```python
from build123d import *

# Parameters (mm, degrees)
SKETCH1_R           = 2.125
BOSS_EXTRUDE1_DEPTH = 5.5
BOSS_EXTRUDE2_START = 7
SKETCH4_R           = 13.5
BOSS_EXTRUDE2_DEPTH = 7
SKETCH6_R           = 11
CUT_EXTRUDE4_DEPTH  = 4
SKETCH5_R           = 1
SKETCH5_R_2         = 1.75
CUT_EXTRUDE2_DEPTH  = 40.376388864
CHAMFER1_SIZE       = 2
SKETCH7_R           = 3
CUT_EXTRUDE5_DEPTH  = 3
FILLET1_R           = 1
SKETCH8_R           = 3
SKETCH8_R_2         = 2.125
BOSS_EXTRUDE3_DEPTH = 0.5
CUT_EXTRUDE6_DEPTH  = 3.25
FILLET2_R           = 0.5


with BuildPart() as part:
    # Sketch1 → Boss-Extrude1 (new body)
    with BuildSketch(Plane.XY):
        with BuildLine():
            Line((-13.071318793, 3.375), (-5.809475019, 31.5))
            ThreePointArc((-5.809475019, 31.5), (0, 36), (5.809475019, 31.5))
            Line((5.809475019, 31.5), (13.071318793, 3.375))
            ThreePointArc((13.071318793, 3.375), (0, -13.5), (-13.071318793, 3.375))
        make_face()
        with Locations((0, 30)):
            Circle(SKETCH1_R, mode=Mode.SUBTRACT)
    extrude(amount=BOSS_EXTRUDE1_DEPTH)

    # Sketch4 → Boss-Extrude2 (add)
    with BuildSketch(Plane(origin=(0, 0, 0), x_dir=(-1, 0, 0), z_dir=(0, 0, -1)).offset(BOSS_EXTRUDE2_START)):
        Circle(SKETCH4_R)
    extrude(amount=-BOSS_EXTRUDE2_DEPTH)

    # Sketch6 → Cut-Extrude4 (cut)
    with BuildSketch(Plane(origin=(0, 0, -7), x_dir=(-1, 0, 0), z_dir=(0, 0, -1))):
        Circle(SKETCH6_R)
    extrude(amount=-CUT_EXTRUDE4_DEPTH, mode=Mode.SUBTRACT)

    # Sketch5 → Cut-Extrude2 (cut, through all)
    with BuildSketch(Plane(origin=(0, 0, -3), x_dir=(-1, 0, 0), z_dir=(0, 0, -1))):
        with Locations((7.42, 0)):
            Circle(SKETCH5_R)
        with Locations((0, -7.42)):
            Circle(SKETCH5_R)
        with Locations((-7.42, 0)):
            Circle(SKETCH5_R)
        with Locations((0, 7.42)):
            Circle(SKETCH5_R)
        Circle(SKETCH5_R_2)
    extrude(amount=-CUT_EXTRUDE2_DEPTH, mode=Mode.SUBTRACT)

    # Chamfer1
    chamfer1_edges = [part.edges().sort_by_distance(p)[0] for p in [
        (9.440396906, 17.4375, 5.5),
        (0, 36, 5.5),
        (-9.440396906, 17.4375, 5.5),
        (0, -13.5, 5.5),
    ]]
    chamfer(chamfer1_edges, length=CHAMFER1_SIZE)

    # Sketch7 → Cut-Extrude5 (cut)
    with BuildSketch(Plane.XY.offset(5.5)):
        Circle(SKETCH7_R)
    extrude(amount=-CUT_EXTRUDE5_DEPTH, mode=Mode.SUBTRACT)

    # Fillet1
    # the kernel refuses this fillet: 1 mm, written as the material it takes off along each edge
    with BuildSketch(Plane(origin=(0, 0, -7), x_dir=(-1, 0, 0), z_dir=(0, -1, 0))) as fillet1_piece_1:
        with BuildLine():
            CenterArc((13.5 - FILLET1_R, -FILLET1_R), FILLET1_R, 0, 90)
            Line((13.5 - FILLET1_R, 0), (13.5, 0))
            Line((13.5, 0), (13.5, -FILLET1_R))
        make_face()
    revolve(axis=Axis((0, 0, -7), (0, 0, -1)), mode=Mode.SUBTRACT)

    # Sketch8 → Boss-Extrude3 (add)
    with BuildSketch(Plane.XY.offset(5.5)):
        with Locations((0, 30)):
            Circle(SKETCH8_R)
        with Locations((0, 30)):
            Circle(SKETCH8_R_2, mode=Mode.SUBTRACT)
    extrude(amount=BOSS_EXTRUDE3_DEPTH)

    # Sketch9 → Cut-Extrude6 (cut)
    with BuildSketch(Plane(origin=(0, 0, 0), x_dir=(-1, 0, 0), z_dir=(0, 0, -1))):
        Polygon((0, 25.669872981), (3.75, 27.834936491), (3.75, 32.165063509), (0, 34.330127019), (-3.75, 32.165063509), (-3.75, 27.834936491), align=None)
    extrude(amount=-CUT_EXTRUDE6_DEPTH, mode=Mode.SUBTRACT)

    # Fillet2
    fillet2_edges = [part.edges().sort_by_distance(p)[0] for p in [
        (1.875, 26.752404736, 0),
        (-1.875, 26.752404736, 0),
        (-3.75, 30, 0),
        (-1.875, 33.247595264, 0),
        (1.875, 33.247595264, 0),
        (3.75, 30, 0),
    ]]
    fillet(fillet2_edges, radius=FILLET2_R)


solid = part.part
```
Work out the finished part from the listing and answer in its coordinate system (mm). A direction names the side the tool comes from. Give positions to 0.01 mm unless a question says otherwise; leave off trailing zeros. Write each loop counter-clockwise with the first axis right and the second up, starting at its lowest first coordinate (ties: lowest second). Pieces come first, ordered by that corner, then holes. Notation, with made-up numbers: (69, -36) -> (112, -36) arc R22 ccw to (112, -21) -> close; hole circle Ø8 at (6, 18). An arc over 180 degrees is marked (long way). Write each question's results on one line, items separated by ' | '.
1. Each of these flat-tipped pins is pushed along its axis until it touches: pin 1 Ø12 at (x, y) = (3, 19.5) entering from -Z; pin 2 Ø2.5 at (x, y) = (7.42, 0) entering from +Z; pin 3 Ø6 at (x, z) = (3.5, 0) entering from -Y. Where does it stop, or does it pass through?
Data:
pin 1: z = 0 | pin 2: z = 5.5 | pin 3: y = -13.49
2. Find section B-B on z = 1.75. Determine the outline of the cut face in (x, y) (3 decimals), and give its area (3 significant figures).
Data:
outline: (-13.071, 3.375) arc R13.5 ccw (long way) to (13.071, 3.375) -> (5.809, 31.5) arc R6 ccw to (-5.809, 31.5) -> close; hole circle Ø2 at (-7.42, 0); hole (-3.75, 27.835) -> (0, 25.67) -> (3.75, 27.835) -> (3.75, 32.165) -> (0, 34.33) -> (-3.75, 32.165) -> close; hole circle Ø3.5 at (0, 0); hole circle Ø2 at (0, -7.42); hole circle Ø2 at (0, 7.42); hole circle Ø2 at (7.42, 0) | area: 875 mm^2
3. Find section D-D on z = -5.25. Determine the outline of the cut face in (x, y).
Data:
outline: circle Ø27 at (0, 0); hole circle Ø22 at (0, 0)
4. Find section C-C on y = 30. Determine the outline of the cut face in (x, z) (3 decimals).
Data:
outline: (-6.197, 0) -> (-4.25, 0) arc R0.5 ccw to (-3.75, 0.5) -> (-3.75, 3.25) -> (-2.125, 3.25) -> (-2.125, 6) -> (-3, 6) -> (-3, 5.5) -> (-4.131, 5.5) -> (-6.197, 3.5) -> close; (2.125, 3.25) -> (3.75, 3.25) -> (3.75, 0.5) arc R0.5 ccw to (4.25, 0) -> (6.197, 0) -> (6.197, 3.5) -> (4.131, 5.5) -> (3, 5.5) -> (3, 6) -> (2.125, 6) -> close
5. Straight lines are drawn through the part: L1, parallel to Y at x = -0.25, z = -4.25; L2, parallel to Y at x = -9, z = -5.75; L3, parallel to X at y = 30, z = 4.8 (3 decimals). For each, find the intervals that lie inside material, in ascending order.
Data:
L1: -13.5 to -11, 11 to 13.5 | L2: -10.06 to -6.32, 6.32 to 10.06 | L3: -4.854 to -2.125, 2.125 to 4.854
6. A tool of negligible diameter and unlimited length cuts with its end or side. For faces 5 (the flat face through (9.4, 17.6, 1.7)), 6 (the flat face through (-3.75, 30, 2)), from which of +Z, -Z, +X, -X, +Y, -Y can it reach the whole face along a straight path? Write none if from no direction.
Data:
face 5: +Z, -Z, +X, +Y | face 6: -Z
7. Determine the mould class of faces 1 (the cylindrical face through (-8.344, -0.383, 1.19)), 2 (the flat face through (-1.901, 33.232, 1.856)), 3 (the flat face through (-8.51, 16.99, 4.51)), 4 (the flat face through (-2, 7, 5.5)) for opening direction X: +X half, -X half, draft (parallel to the pull), parting line (faces both ways), or undercut.
Data:
face 1: undercut | face 2: undercut | face 3: -X half | face 4: draft
8. Find section A-A on y = 0. Determine the outline of the cut face in (x, z), and give its area (3 significant figures).
Data:
outline: (-13.5, -6) arc R1 ccw to (-12.5, -7) -> (-11, -7) -> (-11, -3) -> (-8.42, -3) -> (-8.42, 5.5) -> (-11.5, 5.5) -> (-13.5, 3.5) -> close; (-6.42, -3) -> (-1.75, -3) -> (-1.75, 2.5) -> (-3, 2.5) -> (-3, 5.5) -> (-6.42, 5.5) -> close; (1.75, -3) -> (6.42, -3) -> (6.42, 5.5) -> (3, 5.5) -> (3, 2.5) -> (1.75, 2.5) -> close; (8.42, -3) -> (11, -3) -> (11, -7) -> (12.5, -7) arc R1 ccw to (13.5, -6) -> (13.5, 3.5) -> (11.5, 5.5) -> (8.42, 5.5) -> close | area: 174 mm^2
